```python
from build123d import *

# Parameters (mm, degrees)
SKETCH1_W           = 104
SKETCH1_H           = 95
SKETCH1_R           = 25.5
SKETCH1_R_2         = 2
SKETCH1_W_2         = 9.7
SKETCH1_H_2         = 45.3
BOSS_EXTRUDE1_DEPTH = 4


with BuildPart() as part:
    # Sketch1 → Boss-Extrude1 (new body)
    with BuildSketch(Plane(origin=(0, 0, 0), x_dir=(1, 0, 0), z_dir=(0, 1, 0))):
        with Locations((32.920457223, -35.53611465)):
            Rectangle(SKETCH1_W, SKETCH1_H)
        with Locations(Location((10.920457223, -35.53611465, 0), (0, 0, 270))):
            Circle(SKETCH1_R, mode=Mode.SUBTRACT)
        with Locations(Location((-9.229542777, -15.38611465, 0), (0, 0, 270))):
            Circle(SKETCH1_R_2, mode=Mode.SUBTRACT)
        with Locations(Location((-9.229542777, -55.68611465, 0), (0, 0, 270))):
            Circle(SKETCH1_R_2, mode=Mode.SUBTRACT)
        with Locations(Location((31.070457223, -55.68611465, 0), (0, 0, 270))):
            Circle(SKETCH1_R_2, mode=Mode.SUBTRACT)
        with Locations(Location((31.070457223, -15.38611465, 0), (0, 0, 270))):
            Circle(SKETCH1_R_2, mode=Mode.SUBTRACT)
        with Locations((48.670457223, -35.53611465)):
            Rectangle(SKETCH1_W_2, SKETCH1_H_2, mode=Mode.SUBTRACT)
    extrude(amount=BOSS_EXTRUDE1_DEPTH)


solid = part.part
```
Model file for the job. Use its own axes, mm. A direction names the side the tool comes from. Give positions to 0.01 mm unless a question says otherwise; leave off trailing zeros. Order: outer loops, then holes, each group sorted by start corner. A loop starts at its lowest first (then second) coordinate and runs counter-clockwise, first axis right, second up.
1) 3-axis set-ups, long thin cutter, end or side, ignore diameter. For faces 5 (the flat face through (55, 4, 35)), 6 (the flat face through (49, 2, 58.186)): which of +Z, -Z, +X, -X, +Y, -Y reach the whole face in a straight line?
2) Saw through at B-B, the plane z = 26.5. Write the cut outline in (x, y), then the cut area to 3 significant figures.
3) Saw through at A-A, the plane x = 47.5. Write the cut outline in (y, z).
4) Pin check, flat tips, straight feed: pin 1 (2.5 mm diameter, centred on x = -9.23, z = 15.39, fed in from -Y); pin 2 (6.5 mm diameter, centred on x = 31.07, z = 55.69, fed in from -Y). Stop position of each tip, or through.
5) Mould opens along Z. For faces 1 (the flat face through (43.82, 2, 36)), 2 (the flat face through (-19.08, 2, 36)), 3 (the cylindrical face through (18.58, 1.97, 59.86)), 4 (the flat face through (32, 2, -11.964)) say: +Z half, -Z half, draft (parallel to the pull), parting line (faces both ways), or undercut.
6) Saw through at D-D, the plane y = 0.85. Write the cut outline in (x, z).
7) Saw through at C-C, the plane z = 55. Write the cut outline in (x, y).
8) Wall check: probe 1 along X at (y, z) = (2.65, 45); probe 2 along X at (y, z) = (1.7, 31); probe 3 along Z at (x, y) = (51, 1.2). Give the ranges that are in metal, low to high.
Computed:
1. face 5: +Z, -Z, +X, -X, +Y
1. face 6: +Y, -Y
2. outline: (-19.08, 0) - (-12.92, 0) - (-12.92, 4) - (-19.08, 4) - close; (34.77, 0) - (43.82, 0) - (43.82, 4) - (34.77, 4) - close; (53.52, 0) - (84.92, 0) - (84.92, 4) - (53.52, 4) - close
2. area: 186 mm2
3. outline: (0, -11.96) - (4, -11.96) - (4, 12.89) - (0, 12.89) - close; (0, 58.19) - (4, 58.19) - (4, 83.04) - (0, 83.04) - close
4. pin 1: passes through
4. pin 2: stops at y = 0
5. face 1: undercut
5. face 2: draft
5. face 3: undercut
5. face 4: -Z half
6. outline: (-19.08, -11.96) - (84.92, -11.96) - (84.92, 83.04) - (-19.08, 83.04) - close; hole circle Ø51 at (10.92, 35.54); hole circle Ø4 at (-9.23, 15.39); hole circle Ø4 at (-9.23, 55.69); hole circle Ø4 at (31.07, 15.39); hole circle Ø4 at (31.07, 55.69); hole (43.82, 12.89) - (53.52, 12.89) - (53.52, 58.19) - (43.82, 58.19) - close
7. outline: (-19.08, 0) - (-11.11, 0) - (-11.11, 4) - (-19.08, 4) - close; (-7.35, 0) - (-5.55, 0) - (-5.55, 4) - (-7.35, 4) - close; (27.39, 0) - (29.19, 0) - (29.19, 4) - (27.39, 4) - close; (32.95, 0) - (43.82, 0) - (43.82, 4) - (32.95, 4) - close; (53.52, 0) - (84.92, 0) - (84.92, 4) - (53.52, 4) - close
8. probe 1: x = -19.08 to -12.76, 34.6 to 43.82, 53.52 to 84.92
8. probe 2: x = -19.08 to -14.17, 36.01 to 43.82, 53.52 to 84.92
8. probe 3: z = -11.96 to 12.89, 58.19 to 83.04
